Part print with two shaded views. Sizes in mm from the minimum x, y, z corner. Give positions to 0.01 mm unless a question says otherwise; leave off trailing zeros. Write each loop counter-clockwise with the first axis right and the second up, starting at its lowest first coordinate (ties: lowest second). Pieces come first, ordered by that corner, then holes. Notation, with made-up numbers: (11, -24.5) - (64, -24.5) arc R7 cw to (64, -14.5) - close; hole circle Ø5 at (-33, -6.75). An arc over 180 degrees is marked (long way). One line per item, written item: value. Start each with the question number.
(1) Mould opens along Z. For the marked faces 1, 2, 3 and 4 say: pulls with the +Z half, pulls with the -Z half, needs draft (parallel to the pull), parting line crosses it, or undercut.
(2) Probe L1, parallel to X at y = 32, z = 12.25; L2, parallel to Y at x = 18.5, z = 17.25; L3, parallel to Z at x = 1.5, y = 34.5. List the from-to ranges inside material, lowest first.
(3) Cut at D-D, the plane z = 20.5. List the corners of the cut face in (x, y).
(4) Drop flat-ended pins along their axis: P1, Ø2, axis at x = 18.5, y = 40.5, coming from the -Z side; P2, Ø1.5, axis at x = 4.5, z = 15, coming from the -Y side; P3, Ø4, axis at y = 39.5, z = 9.5, coming from the +X side. Give the stop position or say it passes through.
(5) Cut at A-A, the plane z = 12.2. List the corners of the cut face in (x, y).
(6) Cut at C-C, the plane y = 34.5. List the corners of the cut face in (x, z).
(7) Cut at B-B, the plane x = 12.2. List the corners of the cut face in (y, z).
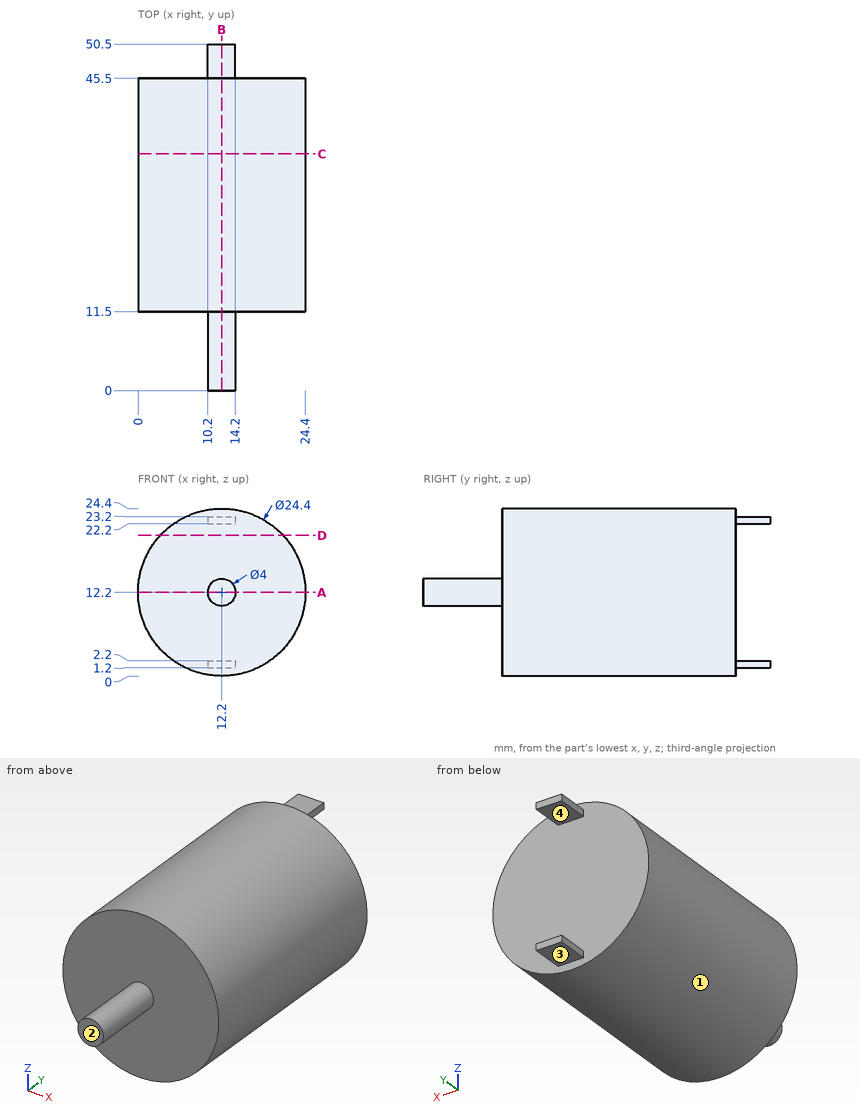
Answers follow:
1. face 1: parting line crosses it
1. face 2: needs draft
1. face 3: pulls with the -Z half
1. face 4: undercut
2. L1: x = 0 to 24.4
2. L2: y = 11.5 to 45.5
2. L3: z = 6.34 to 18.06
3. outline: (3.26, 11.5) - (21.14, 11.5) - (21.14, 45.5) - (3.26, 45.5) - close
4. P1: stops at z = 1.21
4. P2: stops at y = 11.5
4. P3: stops at x = 24.38
5. outline: (0, 11.5) - (10.2, 11.5) - (10.2, 0) - (14.2, 0) - (14.2, 11.5) - (24.4, 11.5) - (24.4, 45.5) - (0, 45.5) - close
6. outline: circle Ø24.4 at (12.2, 12.2)
7. outline: (0, 10.2) - (11.5, 10.2) - (11.5, 0) - (45.5, 0) - (45.5, 1.2) - (50.5, 1.2) - (50.5, 2.2) - (45.5, 2.2) - (45.5, 22.2) - (50.5, 22.2) - (50.5, 23.2) - (45.5, 23.2) - (45.5, 24.4) - (11.5, 24.4) - (11.5, 14.2) - (0, 14.2) - close
